CAD build for the part. Positions are in the model's coordinates, mm. Coordinates: 2 decimals unless noted, no trailing zeros. Order: outer loops, then holes, each group sorted by start corner. A loop starts at its lowest first (then second) coordinate and runs counter-clockwise, first axis right, second up. Notation, with made-up numbers: M 23,-11.5 L 64,-11.5 A19 ccw 64,21.5 Z; hole C 15,62 d9. An arc over 180 degrees is marked long. One line per item, written item: value.
from build123d import *

# Parameters (mm, degrees)
SKETCH1_W           = 200
SKETCH1_H           = 2400
BOSS_EXTRUDE1_DEPTH = 80
CHAMFER1_SIZE       = 25
SKETCH2_W           = 130
SKETCH2_H           = 2400
CUT_EXTRUDE1_DEPTH  = 16.51744982


with BuildPart() as part:
    # Sketch1 → Boss-Extrude1 (new body)
    with BuildSketch(Plane(origin=(0, 0, 0), x_dir=(1, 0, 0), z_dir=(0, 1, 0))):
        Rectangle(SKETCH1_W, SKETCH1_H)
    extrude(amount=BOSS_EXTRUDE1_DEPTH)

    # Chamfer1
    chamfer1_edges = [part.edges().sort_by_distance(p)[0] for p in [
        (-100, 0, 0),
        (100, 0, 0),
    ]]
    chamfer(chamfer1_edges, length=CHAMFER1_SIZE)

    # Sketch2 → Cut-Extrude1 (cut)
    with BuildSketch(Plane(origin=(0, 80, 0), x_dir=(1, 0, 0), z_dir=(0, 1, 0))):
        Rectangle(SKETCH2_W, SKETCH2_H)
    extrude(amount=-CUT_EXTRUDE1_DEPTH, mode=Mode.SUBTRACT)


solid = part.part
Q1. Slice it at B-B (x = 1). List the corners of the cut face in (y, z).
Recorded:
outline: M 0,-1200 L 63.48,-1200 L 63.48,1200 L 0,1200 Z
Q2. Drill centre lines: line 1 along X through (y, z) = (68, -721); line 2 along Y through (x, z) = (34, -581); line 3 along X through (y, z) = (6.5, 737). Where is each one in solid material? Low to high.
Recorded:
line 1: x = -100 to -65, 65 to 100
line 2: y = 0 to 63.48
line 3: x = -81.5 to 81.5
Q3. Pin check, flat tip, straight feed: pin 1 Ø1 at (x, z) = (-60, 485.5) entering from +Y. Stop position of the tip, or through.
Recorded:
pin 1: stops at y = 63.48
Q4. Mould opens along Z. For faces 1 (the face through (-1, 39, 1200)), 2 (the face through (-1, 39, -1200)), 3 (the face through (-1, 63.483, -17)) say: released by +Z, released by -Z, zero draft, split by the parting line, or undercut.
Recorded:
face 1: released by +Z
face 2: released by -Z
face 3: zero draft
Q5. Slice it at A-A (z = -303). List the corners of the cut face in (x, y).
Recorded:
outline: M -100,25 L -75,0 L 75,0 L 100,25 L 100,80 L 65,80 L 65,63.48 L -65,63.48 L -65,80 L -100,80 Z
